Could you check a few things on this model? Use its own coordinates, in mm. Round coordinates to 2 decimals unless told otherwise and drop trailing zeros. Write each loop counter-clockwise with the first axis right and the second up, starting at its lowest first coordinate (ties: lowest second). Pieces come first, ordered by that corner, then holes. Notation, with made-up numbers: (48.25, 9.25) -> (56.25, 9.25) arc R20 ccw to (56.25, 21.25) -> close; hole circle Ø7 at (54.25, 24.5). An arc over 180 degrees is marked (long way). Answer in a Markdown table with one row per item. Add a question column.
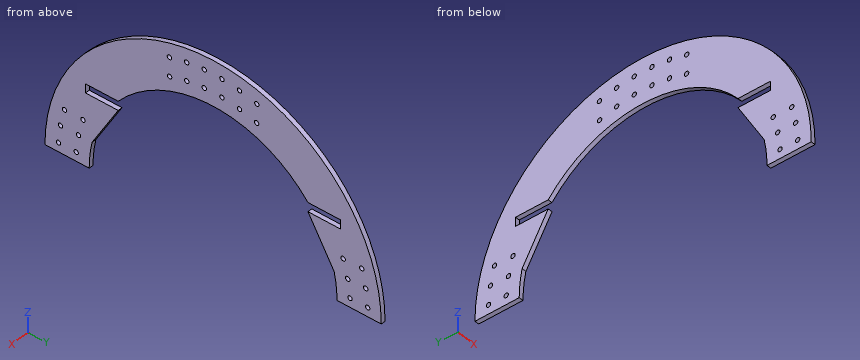
Autodesk Inventor part; units mm, degrees
ref_plane "YZ Plane" through (0, 0, 0) normal (1, 0, 0) x (0, 1, 0)
ref_plane "XZ Plane" through (0, 0, 0) normal (0, 1, 0) x (-1, 0, 0)
ref_plane "XY Plane" through (0, 0, 0) normal (0, 0, 1) x (1, 0, 0)
sketch "Sketch1" plane through (0, 0, 0) normal (1, 0, 0) x (0, 1, 0)
  arc A0 (241.3, 0) -> (-241.3, 0) centre (0, 0) ccw
  arc A1 (177.8, 0) -> (-177.8, 0) centre (0, 0) ccw
  line L0 (-177.8, 0) -> (-241.3, 0)
  circle A2 centre (221.8868, 12.7) radius 3.175
  circle A3 centre (0, 0) radius 222.25 construction
  circle A4 centre (218.9887, 37.9341) radius 3.175
  circle A5 centre (213.2304, 62.6728) radius 3.175
  circle A6 centre (0, 0) radius 196.85 construction
  circle A7 centre (186.6826, 62.4463) radius 3.175
  circle A8 centre (193.1693, 37.8886) radius 3.175
  circle A9 centre (196.4399, 12.7) radius 3.175
  line L1 (0, 0) -> (360.6027, 0)
  line L2 (360.6027, 0) -> (-412.5993, 0)
  line L3 (0, 0) -> (0, -65.1131)
  circle A10 centre (-221.8868, 12.7) radius 3.175
  circle A11 centre (-218.9887, 37.9341) radius 3.175
  circle A12 centre (-213.2304, 62.6728) radius 3.175
  circle A13 centre (-186.6826, 62.4463) radius 3.175
  circle A14 centre (-193.1693, 37.8886) radius 3.175
  circle A15 centre (-196.4399, 12.7) radius 3.175
  line L4 (0, 0) -> (205.1572, 205.1572)
  line L5 (0, 0) -> (-243.5425, 243.5425)
  circle A16 centre (-12.7, 221.8868) radius 3.175
  circle A17 centre (-37.9341, 218.9887) radius 3.175
  circle A18 centre (-62.6728, 213.2304) radius 3.175
  circle A19 centre (-62.4463, 186.6826) radius 3.175
  circle A20 centre (-37.8886, 193.1693) radius 3.175
  circle A21 centre (-12.7, 196.4399) radius 3.175
  circle A22 centre (12.7, 221.8868) radius 3.175
  circle A23 centre (37.9341, 218.9887) radius 3.175
  circle A24 centre (62.6728, 213.2304) radius 3.175
  circle A25 centre (62.4463, 186.6826) radius 3.175
  circle A26 centre (37.8886, 193.1693) radius 3.175
  circle A27 centre (12.7, 196.4399) radius 3.175
  line L6 (241.3, 0) -> (177.8, 0)
  dimension "d0" = 482.6
  dimension "d1" = 355.6
  dimension "d2" = 6.35
  dimension "d3" = 444.5
  dimension "d4" = 6.35
  dimension "d5" = 6.35
  dimension "d6" = 25.4
  dimension "d7" = 25.4
  dimension "d8" = 393.7
  dimension "d9" = 6.35
  dimension "d10" = 6.35
  dimension "d11" = 6.35
  dimension "d13" = 12.7
  dimension "d14" = 12.7
  dimension "d15" = 25.4
  dimension "d16" = 25.4
  dimension "d17" = 45
  dimension "d18" = 45
extrude "Extrusion1" add sketch "Sketch1" along normal blind 6.35 contours L1 A1 L4 A0 | L4 A1 L5 A0 | L5 A1 L0 A0
sketch "Sketch2" plane through (6.35, 0, 0) normal (1, 0, 0) x (0, 0, -1)
  line L0 (-101.6, 183.162) -> (-101.6, 145.9119)
  arc A0 (101.6, 145.9119) -> (-101.6, 145.9119) centre (0, 0) ccw
  line L1 (101.6, 145.9119) -> (101.6, 183.162)
  line L2 (101.6, 183.162) -> (114.3, 183.162)
  line L3 (114.3, 183.162) -> (114.3, 136.1923)
  arc A1 (177.8, 0) -> (114.3, 136.1923) centre (0, 0) ccw
  line L4 (177.8, 0) -> (254, 0)
  arc A2 (254, 0) -> (50.0287, 249.0244) centre (0, 0) ccw
  arc A3 (36.5783, 256.4729) -> (50.0287, 249.0244) centre (55.0316, 273.9268) ccw
  arc A4 (36.5783, 256.4729) -> (-36.5783, 256.4729) centre (0, 221.8757) ccw
  arc A5 (-50.0287, 249.0244) -> (-36.5783, 256.4729) centre (-55.0316, 273.9268) ccw
  arc A6 (-50.0287, 249.0244) -> (-254, 0) centre (0, 0) ccw
  line L5 (-254, 0) -> (-177.8, 0)
  arc A7 (-114.3, 136.1923) -> (-177.8, 0) centre (0, 0) ccw
  line L6 (-114.3, 136.1923) -> (-114.3, 183.162)
  line L7 (-114.3, 183.162) -> (-101.6, 183.162)
  circle A8 centre (-196.4399, 12.7) radius 3.302
  circle A9 centre (-218.9887, 37.9341) radius 3.302
  circle A10 centre (-186.6826, 62.4463) radius 3.302
  circle A11 centre (-62.4463, 186.6826) radius 3.302
  circle A12 centre (-37.9341, 218.9887) radius 3.302
  circle A13 centre (-12.7, 196.4399) radius 3.302
  circle A14 centre (12.7, 221.8868) radius 3.302
  circle A15 centre (37.8886, 193.1693) radius 3.302
  circle A16 centre (62.6728, 213.2304) radius 3.302
  circle A17 centre (196.4399, 12.7) radius 3.302
  circle A18 centre (193.1693, 37.8886) radius 3.302
  circle A19 centre (186.6826, 62.4463) radius 3.302
  circle A20 centre (213.2304, 62.6728) radius 3.302
  circle A21 centre (218.9887, 37.9341) radius 3.302
  circle A22 centre (221.8868, 12.7) radius 3.302
  circle A23 centre (62.4463, 186.6826) radius 3.302
  circle A24 centre (37.9341, 218.9887) radius 3.302
  circle A25 centre (12.7, 196.4399) radius 3.302
  circle A26 centre (-12.7, 221.8868) radius 3.302
  circle A27 centre (-37.8886, 193.1693) radius 3.302
  circle A28 centre (-62.6728, 213.2304) radius 3.302
  circle A29 centre (-213.2304, 62.6728) radius 3.302
  circle A30 centre (-193.1693, 37.8886) radius 3.302
  circle A31 centre (-221.8868, 12.7) radius 3.302
  circle A32 centre (0, 259.6856) radius 3.302
  line L8 (0, 0) -> (-75.0645, 0)
  line L9 (-114.3, 183.162) -> (-101.6, 183.162)
  line L10 (-101.6, 183.162) -> (-101.6, 75.1342)
  line L11 (-101.6, 75.1342) -> (-114.3, 75.1342)
  line L12 (-114.3, 75.1342) -> (-114.3, 183.162)
  line L13 (-114.3, -136.1923) -> (-114.3, -183.162)
  line L14 (-114.3, -183.162) -> (-101.6, -183.162)
  line L15 (-101.6, -183.162) -> (-101.6, -75.1342)
  line L16 (-101.6, -75.1342) -> (-114.3, -75.1342)
  line L17 (-114.3, -75.1342) -> (-114.3, -183.162)
  line L18 (-114.3, -183.162) -> (-101.6, -183.162)
  line L19 (-101.6, -183.162) -> (-101.6, -75.1342)
  line L20 (-101.6, -75.1342) -> (-114.3, -75.1342)
  line L21 (-114.3, -75.1342) -> (-114.3, -183.162)
  point P0 (0, 0)
extrude "Extrusion2" cut sketch "Sketch2" against normal blind 25.4 contours L0 L10 L11 L12 L6 L7 | L17 L16 L15 L14 L13
sketch "Sketch3" plane through (6.35, 0, 0) normal (1, 0, 0) x (0, 0, -1)
  line L0 (-101.6, 183.162) -> (-101.6, 136.1923)
  line L1 (-101.6, 136.1923) -> (-38.1, 173.6699)
  arc A0 (38.1, 173.6699) -> (-38.1, 173.6699) centre (0, 0) ccw
  line L2 (38.1, 173.6699) -> (101.6, 136.1923)
  line L3 (101.6, 136.1923) -> (101.6, 183.162)
  line L4 (101.6, 183.162) -> (114.3, 183.162)
  line L5 (114.3, 183.162) -> (114.3, 136.1923)
  arc A1 (177.8, 0) -> (114.3, 136.1923) centre (0, 0) ccw
  line L6 (177.8, 0) -> (254, 0)
  arc A2 (254, 0) -> (50.0287, 249.0244) centre (0, 0) ccw
  arc A3 (36.5783, 256.4729) -> (50.0287, 249.0244) centre (55.0316, 273.9268) ccw
  arc A4 (36.5783, 256.4729) -> (-36.5783, 256.4729) centre (0, 221.8757) ccw
  arc A5 (-50.0287, 249.0244) -> (-36.5783, 256.4729) centre (-55.0316, 273.9268) ccw
  arc A6 (-50.0287, 249.0244) -> (-254, 0) centre (0, 0) ccw
  line L7 (-254, 0) -> (-177.8, 0)
  arc A7 (-114.3, 136.1923) -> (-177.8, 0) centre (0, 0) ccw
  line L8 (-114.3, 136.1923) -> (-114.3, 183.162)
  line L9 (-114.3, 183.162) -> (-101.6, 183.162)
  circle A8 centre (-196.4399, 12.7) radius 3.302
  circle A9 centre (-218.9887, 37.9341) radius 3.302
  circle A10 centre (-186.6826, 62.4463) radius 3.302
  circle A11 centre (-62.4463, 186.6826) radius 3.302
  circle A12 centre (-37.9341, 218.9887) radius 3.302
  circle A13 centre (-12.7, 196.4399) radius 3.302
  circle A14 centre (12.7, 221.8868) radius 3.302
  circle A15 centre (37.8886, 193.1693) radius 3.302
  circle A16 centre (62.6728, 213.2304) radius 3.302
  circle A17 centre (196.4399, 12.7) radius 3.302
  circle A18 centre (193.1693, 37.8886) radius 3.302
  circle A19 centre (186.6826, 62.4463) radius 3.302
  circle A20 centre (213.2304, 62.6728) radius 3.302
  circle A21 centre (218.9887, 37.9341) radius 3.302
  circle A22 centre (221.8868, 12.7) radius 3.302
  circle A23 centre (62.4463, 186.6826) radius 3.302
  circle A24 centre (37.9341, 218.9887) radius 3.302
  circle A25 centre (12.7, 196.4399) radius 3.302
  circle A26 centre (-12.7, 221.8868) radius 3.302
  circle A27 centre (-37.8886, 193.1693) radius 3.302
  circle A28 centre (-62.6728, 213.2304) radius 3.302
  circle A29 centre (-213.2304, 62.6728) radius 3.302
  circle A30 centre (-193.1693, 37.8886) radius 3.302
  circle A31 centre (-221.8868, 12.7) radius 3.302
  circle A32 centre (0, 259.6856) radius 3.302
  line L10 (0, 0) -> (-50.0287, 0)
  arc A33 (0, 177.8) -> (-101.6, 145.9119) centre (0, 0) ccw
  arc A34 (-38.1, 173.6699) -> (-101.6, 145.9119) centre (0, 0) ccw
  line L11 (-101.6, -145.9119) -> (-101.6, -183.162)
  line L12 (-101.6, -183.162) -> (-114.3, -183.162)
  line L13 (-114.3, -183.162) -> (-114.3, -136.1923)
  arc A35 (-177.8, 0) -> (-114.3, -136.1923) centre (0, 0) ccw
  line L14 (-177.8, 0) -> (-254, 0)
  line L15 (-254, 0) -> (-254, -254)
  line L16 (-254, -254) -> (254, -254)
  line L17 (254, -254) -> (254, 0)
  line L18 (254, 0) -> (177.8, 0)
  arc A36 (114.3, -136.1923) -> (177.8, 0) centre (0, 0) ccw
  line L19 (114.3, -136.1923) -> (114.3, -183.162)
  line L20 (114.3, -183.162) -> (101.6, -183.162)
  line L21 (101.6, -183.162) -> (101.6, -145.9119)
  arc A37 (-101.6, -145.9119) -> (101.6, -145.9119) centre (0, 0) ccw
  circle A38 centre (221.8868, -12.7) radius 3.302
  circle A39 centre (193.1693, -37.8886) radius 3.302
  circle A40 centre (213.2304, -62.6728) radius 3.302
  circle A41 centre (62.4463, -186.6826) radius 3.302
  circle A42 centre (37.9341, -218.9887) radius 3.302
  circle A43 centre (12.7, -221.8868) radius 3.302
  circle A44 centre (-12.7, -221.8868) radius 3.302
  circle A45 centre (-37.9341, -218.9887) radius 3.302
  circle A46 centre (-62.6728, -213.2304) radius 3.302
  circle A47 centre (-186.6826, -62.4463) radius 3.302
  circle A48 centre (-218.9887, -37.9341) radius 3.302
  circle A49 centre (-196.4399, -12.7) radius 3.302
  circle A50 centre (-221.8868, -12.7) radius 3.302
  circle A51 centre (-193.1693, -37.8886) radius 3.302
  circle A52 centre (-213.2304, -62.6728) radius 3.302
  circle A53 centre (-62.4463, -186.6826) radius 3.302
  circle A54 centre (-37.8886, -193.1693) radius 3.302
  circle A55 centre (-12.7, -196.4399) radius 3.302
  circle A56 centre (12.7, -196.4399) radius 3.302
  circle A57 centre (37.8886, -193.1693) radius 3.302
  circle A58 centre (62.6728, -213.2304) radius 3.302
  circle A59 centre (186.6826, -62.4463) radius 3.302
  circle A60 centre (218.9887, -37.9341) radius 3.302
  circle A61 centre (196.4399, -12.7) radius 3.302
  circle A62 centre (-215.9, -215.9) radius 3.302
  circle A63 centre (215.9, -215.9) radius 3.302
  line L22 (-101.6, -136.1923) -> (-38.1, -173.6699)
  line L23 (-101.6, -183.162) -> (-101.6, -145.9119)
  line L24 (-101.6, -136.1923) -> (-101.6, -145.9119)
  arc A64 (-101.6, -145.9119) -> (0, -177.8) centre (0, 0) ccw
  arc A65 (-101.6, -145.9119) -> (-38.1, -173.6699) centre (0, 0) ccw
extrude "Extrusion3" add sketch "Sketch3" against normal blind 6.35 contours A33 L1 L0 | L24 L22 A37
properties part number "19in inner coil" material "Acetal Resin, Black"
(1) Suppose I cut it at D-D, the plane y = -81. Please give me the cut outline in (x, z), then the cut area to 3 significant figures.
(2) I need wall thicknesses on L1, parallel to Y at x = 2, z = 11.5; L2, parallel to Y at x = 2, z = 184.5; L3, parallel to Y at x = 1.75, z = 62. Which ranges of each line are inside material? Lowest first, please.
(3) Suppose I cut it at B-B, the plane y = 0. Please give me the cut outline in (x, z), then the cut area to 3 significant figures.
(4) Suppose I cut it at C-C, the plane x = 3.5. State how many separate pieces and enclosed holes the cut face has, then the cut area to 3 significant figures.
(5) For P1, Ø1, axis at x = 2.5, z = 159, coming from the -Y side; P2, Ø5.5, axis at y = 221.89, z = 12.7, coming from the -X side; P3, Ø1.5, axis at x = 2.5, z = 48, coming from the +Y side; P4, Ø1, axis at x = 2.5, y = 177, coming from the +Z side, each with a flat end and sliding along its axis, tell me the tip position at first contact or that it passes through.
(6) Suppose I cut it at A-A, the plane y = 166. Please give me the cut outline in (x, z).
Response:
| question | item | result |
|---|---|---|
| 1 | outline | (0, 158.28) -> (6.35, 158.28) -> (6.35, 227.3) -> (0, 227.3) -> close |
| 1 | area | 438 mm² |
| 2 | L1 | -241.03 to -224.83, -218.95 to -199.38, -193.5 to -177.43, 177.43 to 193.5, 199.38 to 218.95, 224.83 to 241.03 |
| 2 | L2 | -155.52 to -64.75, -60.14 to 60.14, 64.75 to 155.52 |
| 2 | L3 | -233.2 to -216.33, -210.13 to -189.83, -183.54 to -159.56, 159.56 to 183.54, 189.83 to 210.13, 216.33 to 233.2 |
| 3 | outline | (0, 177.8) -> (6.35, 177.8) -> (6.35, 241.3) -> (0, 241.3) -> close |
| 3 | area | 403 mm² |
| 4 | separate pieces | 1 |
| 4 | enclosed holes | 24 |
| 4 | area | 40,900 mm² |
| 5 | P1 | y = -181.94 |
| 5 | P2 | through |
| 5 | P3 | y = 236.63 |
| 5 | P4 | z = 164.54 |
| 6 | outline | (0, 51.1) -> (6.35, 51.1) -> (6.35, 101.6) -> (0, 101.6) -> close; (0, 114.3) -> (6.35, 114.3) -> (6.35, 175.13) -> (0, 175.13) -> close |
